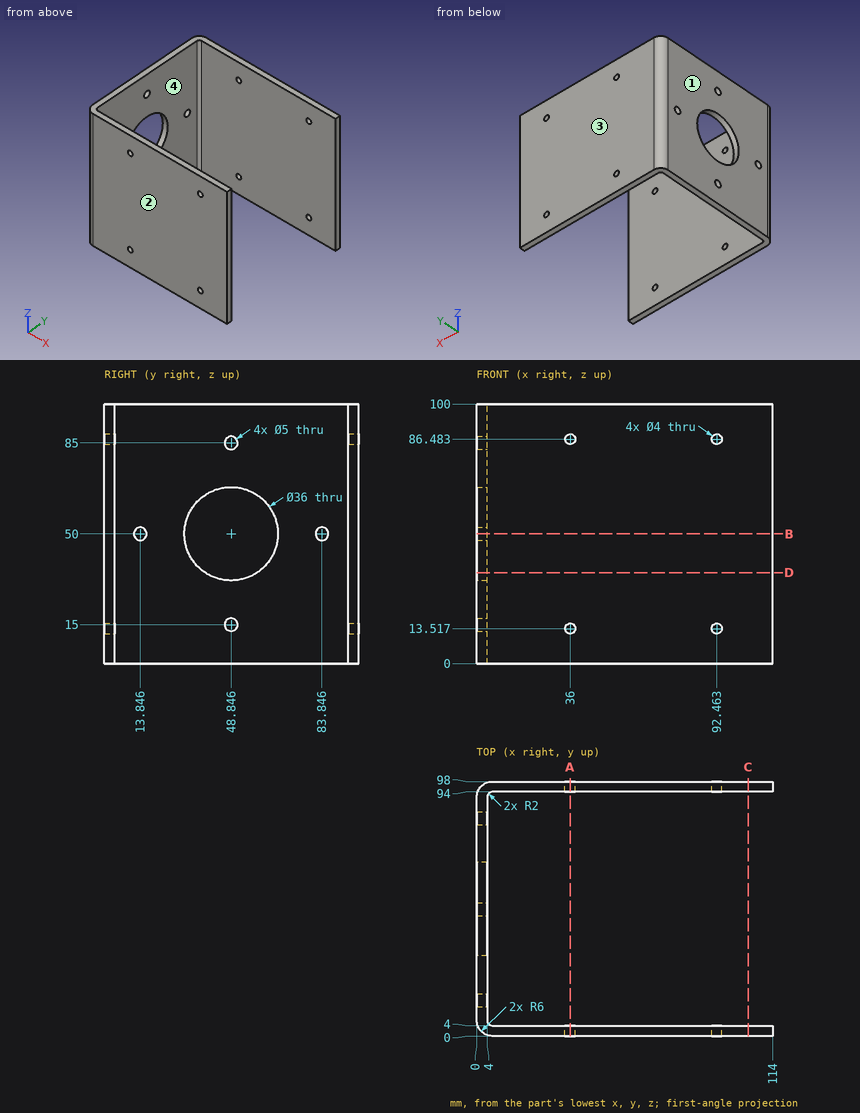
Can you work these out from the drawing? Everything is in mm from the part's minimum corner. Give positions to 0.01 mm unless a question says otherwise; leave off trailing zeros. Write each loop counter-clockwise with the first axis right and the second up, starting at its lowest first coordinate (ties: lowest second). Pieces come first, ordered by that corner, then holes. Notation, with made-up numbers: (13, -9.75) -> (70, -9.75) arc R20 cw to (70, 10.25) -> close; hole circle Ø9 at (41, 14.25). An arc over 180 degrees is marked (long way). Write each question's results on one line, items separated by ' | '.
Item 1: For pin 1 Ø6 at (y, z) = (73, 45) entering from -X; pin 2 Ø1 at (y, z) = (54.5, 75) entering from +X, each with a flat end and sliding along its axis, tell me the tip position at first contact or that it passes through.
Output:
pin 1: stops at x = 0 | pin 2: stops at x = 4
Item 2: If I drill on L1, parallel to Z at x = 36, y = 1; L2, parallel to Y at x = 55, z = 52.5; L3, parallel to Y at x = 1.25, z = 50 (1 decimal), over which ranges is the centre line in solid material (lowest first)?
Output:
L1: z = 0 to 11.52, 15.52 to 84.48, 88.48 to 100 | L2: y = 0 to 4, 94 to 98 | L3: y = 2.3 to 11.3, 16.3 to 30.8, 66.8 to 81.3, 86.3 to 95.7
Item 3: Suppose I cut it at B-B on z = 50. Write out the boundary of the cut face in (x, y), plus the area to 3 significant figures.
Output:
outline: (0, 6) arc R6 ccw to (6, 0) -> (114, 0) -> (114, 4) -> (6, 4) arc R2 cw to (4, 6) -> (4, 11.35) -> (0, 11.35) -> close; (0, 16.35) -> (4, 16.35) -> (4, 30.85) -> (0, 30.85) -> close; (0, 66.85) -> (4, 66.85) -> (4, 81.35) -> (0, 81.35) -> close; (0, 86.35) -> (4, 86.35) -> (4, 92) arc R2 cw to (6, 94) -> (114, 94) -> (114, 98) -> (6, 98) arc R6 ccw to (0, 92) -> close | area: 1,070 mm^2
Item 4: Suppose I cut it at D-D on z = 35. Write out the boundary of the cut face in (x, y), plus the area to 3 significant figures.
Output:
outline: (0, 6) arc R6 ccw to (6, 0) -> (114, 0) -> (114, 4) -> (6, 4) arc R2 cw to (4, 6) -> (4, 38.9) -> (0, 38.9) -> close; (0, 58.8) -> (4, 58.8) -> (4, 92) arc R2 cw to (6, 94) -> (114, 94) -> (114, 98) -> (6, 98) arc R6 ccw to (0, 92) -> close | area: 1,180 mm^2
Item 5: We'd pull the mould along Y, two halves only. Please class the marked faces 1, 2, 3 and 4: pulls with the +Y half, pulls with the -Y half, needs draft (parallel to the pull), parting line crosses it, or undercut.
Output:
face 1: needs draft | face 2: pulls with the -Y half | face 3: pulls with the +Y half | face 4: undercut
Item 6: Suppose I cut it at C-C on x = 104.5. Write out the boundary of the cut face in (y, z).
Output:
outline: (0, 0) -> (4, 0) -> (4, 100) -> (0, 100) -> close; (94, 0) -> (98, 0) -> (98, 100) -> (94, 100) -> close
Item 7: Suppose I cut it at A-A on x = 36. Write out the boundary of the cut face in (y, z).
Output:
outline: (0, 0) -> (4, 0) -> (4, 11.52) -> (0, 11.52) -> close; (0, 15.52) -> (4, 15.52) -> (4, 84.48) -> (0, 84.48) -> close; (0, 88.48) -> (4, 88.48) -> (4, 100) -> (0, 100) -> close; (94, 0) -> (98, 0) -> (98, 11.52) -> (94, 11.52) -> close; (94, 15.52) -> (98, 15.52) -> (98, 84.48) -> (94, 84.48) -> close; (94, 88.48) -> (98, 88.48) -> (98, 100) -> (94, 100) -> close
